Geometry check sheet. Reference: drawing and pictorial views, mm from the part's lowest x, y, z. A direction names the side the tool comes from. Round coordinates to 2 decimals unless told otherwise and drop trailing zeros. Order: outer loops, then holes, each group sorted by start corner. A loop starts at its lowest first (then second) coordinate and runs counter-clockwise, first axis right, second up.
(1) Sectioned sample at B-B (y = 19.25). Record the boundary of the cut face in (x, z), plus the area to 3 significant figures.
(2) Material ranges on line 1 along X through (y, z) = (4, 7.5); line 2 along Z through (x, y) = (23, 16); line 3 along Y through (x, z) = (1, 60), recorded low to high.
(3) Release check for a two-part mould opening along X. For the marked faces 1, 2 and 3 record: +X half, -X half, draft (parallel to the pull), parting line (faces both ways), or undercut.
(4) Go/stop test with flat-tipped pins: pin 1 (2.5 mm diameter, centred on y = 12.5, z = 46.5, fed in from -X); pin 2 (6 mm diameter, centred on x = 34.5, y = 4, fed in from +Z). Record where each tip stops, or that it passes through.
(5) Sectioned sample at A-A (z = 31). Record the boundary of the cut face in (x, y).
(6) Sectioned sample at D-D (x = 9). Record the boundary of the cut face in (y, z).
(7) Sectioned sample at C-C (z = 46.5). Record the boundary of the cut face in (x, y).
(8) Set-up check for the marked faces 4 and 5: record each of +Z, -Z, +X, -X, +Y, -Y from which the full face is reachable in a straight line by a thin tool's end or side.
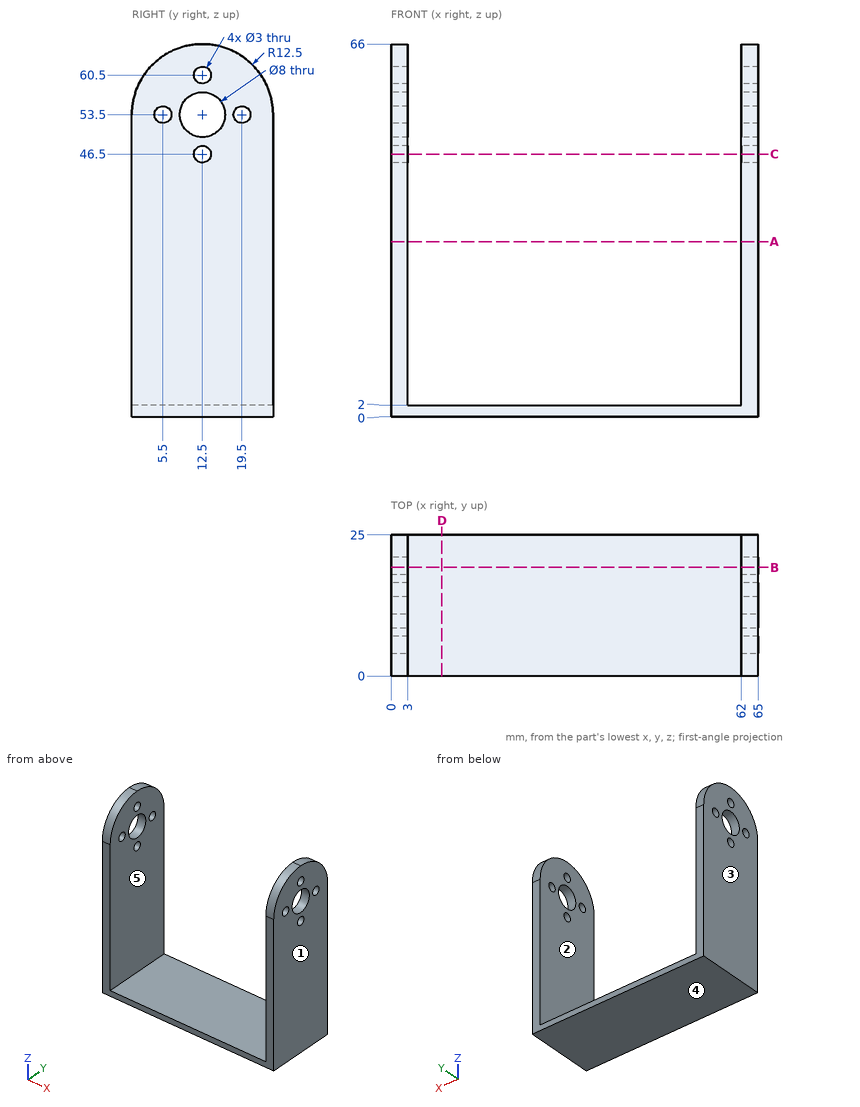
Answer below:
1. outline: (0, 0) - (65, 0) - (65, 52.02) - (62, 52.02) - (62, 2) - (3, 2) - (3, 52.02) - (0, 52.02) - close; (0, 54.98) - (3, 54.98) - (3, 64.02) - (0, 64.02) - close; (62, 54.98) - (65, 54.98) - (65, 64.02) - (62, 64.02) - close
1. area: 484 mm2
2. line 1: x = 0 to 3, 62 to 65
2. line 2: z = 0 to 2
2. line 3: y = 1.82 to 11.09, 13.91 to 23.18
3. face 1: +X half
3. face 2: undercut
3. face 3: -X half
4. pin 1: passes through
4. pin 2: stops at z = 2
5. outline: (0, 0) - (3, 0) - (3, 25) - (0, 25) - close; (62, 0) - (65, 0) - (65, 25) - (62, 25) - close
6. outline: (0, 0) - (25, 0) - (25, 2) - (0, 2) - close
7. outline: (0, 0) - (3, 0) - (3, 11) - (0, 11) - close; (0, 14) - (3, 14) - (3, 25) - (0, 25) - close; (62, 0) - (65, 0) - (65, 11) - (62, 11) - close; (62, 14) - (65, 14) - (65, 25) - (62, 25) - close
8. face 4: -Z, +X, -X, +Y, -Y
8. face 5: +Z, +Y, -Y
